from build123d import *

# Parameters (mm, degrees)
F1_DEPTH  = 5.2959
F2_DEPTH  = 41.276
F4_DEPTH  = 3.7084
F12_DEPTH = 3.7084
F6_DEPTH  = 10.5918
F7_DEPTH  = 41.276
F8_W      = 3.5700032353
F8_H      = 0.1361034085
F8_H_2    = 4.0928895229
F8_H_3    = 0.1088827268
F8_H_4    = 4.1201102046
F8_H_5    = 0.0816620451
F8_H_6    = 4.1473308863
F8_H_7    = 0.0544413634
F8_H_8    = 4.174551568
F8_H_9    = 0.0272206817
F8_H_10   = 4.2017722497
F8_H_11   = 4.2289929314
F14_DEPTH = 12.7
F9_R      = 1.016


with BuildPart() as f1:
    # F0 (on Right) → F1 (new body, symmetric)
    with BuildSketch(Plane.YZ):
        Polygon((25.4, 38.1), (0, 0), (41.275, 0), (41.275, 7.9375), (25.4, 15.875), align=None)
    extrude(amount=F1_DEPTH, both=True)

    # F10 (on Front) → F2 (cut, through all)
    with BuildSketch(Plane.XZ):
        with BuildLine():
            Line((-1.5875, 14.8209), (-5.2959, 14.8209))
            Line((-5.2959, 14.8209), (-5.2959, 5.2959000144))
            ThreePointArc((-5.2959, 5.2959000144), (-4.2692972482, 8.4295333251), (-1.5875, 10.3482658379))
            Line((-1.5875, 10.3482658379), (-1.5875, 14.8209))
        make_face()
        with BuildLine():
            Line((5.2959, 5.2959), (5.2959, 14.8209))
            Line((5.2959, 14.8209), (1.5875, 14.8209))
            Line((1.5875, 14.8209), (1.5875, 10.3482658379))
            ThreePointArc((1.5875, 10.3482658379), (4.2692972525, 8.4295333193), (5.2959, 5.2959))
        make_face()
        with BuildLine():
            ThreePointArc((0, 0), (-3.7447668076, 1.5511332026), (-5.2959, 5.2959000144))
            Line((-5.2959, 5.2959000144), (-5.2959, 0))
            Line((-5.2959, 0), (0, 0))
        make_face()
        with BuildLine():
            ThreePointArc((5.2959, 5.2959), (3.7447668025, 1.5511331975), (0, 0))
            Line((0, 0), (5.2959, 0))
            Line((5.2959, 0), (5.2959, 5.2959))
        make_face()
    extrude(amount=-F2_DEPTH, mode=Mode.SUBTRACT)

    # F3 (on face) → F4 (cut)
    with BuildSketch(Plane.YZ.offset(5.2959)):
        Polygon((17.4625, 14.8209), (27.5082, 14.8209), (25.4, 15.875), (25.4, 19.5834), align=None)
    extrude(amount=-F4_DEPTH, mode=Mode.SUBTRACT)

    # F11 (on face) → F12 (cut)
    with BuildSketch(Plane(origin=(-5.2959, 0, 0), x_dir=(0, -1, 0), z_dir=(-1, 0, 0))):
        Polygon((-27.5082, 14.8209), (-17.4625, 14.8209), (-25.4, 19.5834), (-25.4, 15.875), align=None)
    extrude(amount=-F12_DEPTH, mode=Mode.SUBTRACT)

    # F5 (on face) → F6 (join)
    with BuildSketch(Plane.YZ.offset(5.2959)):
        with BuildLine():
            add(Edge.make_bspline(
                [(9.8806, 14.8209), (9.7887178245, 17.0000575052), (7.8190504565, 20.9662638554), (18.9792610557, 30.802658642), (25.4, 38.1)],
                knots=[0, 0, 0, 0, 0.3217761524, 1, 1, 1, 1], degree=3))
            Line((9.8806, 14.8209), (25.4, 38.1))
        make_face()
    extrude(amount=-F6_DEPTH)

    # F13 (on Front) → F7 (cut, through all)
    with BuildSketch(Plane.XZ):
        with BuildLine():
            add(Edge.make_bspline(
                [(-5.2959, 14.8209), (-5.2959, 15.5472858351), (-5.2959, 17.5957404535), (-5.2959, 22.9229933342), (-5.2959, 29.9563074991), (-5.2959, 35.6675528807), (-5.2959, 38.1)],
                knots=[0, 0, 0, 0, 2.1791575052, 6.1453638554, 15.981758642, 23.2791, 23.2791, 23.2791, 23.2791], degree=3))
            Line((-5.2959, 14.8209), (-2.38125, 38.1))
            Line((-2.38125, 38.1), (-5.2959, 38.1))
        make_face()
        with BuildLine():
            Line((2.38125, 38.1), (5.2959, 14.8209))
            add(Edge.make_bspline(
                [(5.2959, 14.8209), (5.2959, 15.5472858351), (5.2959, 17.5957404535), (5.2959, 22.9229933342), (5.2959, 29.9563074991), (5.2959, 35.6675528807), (5.2959, 38.1)],
                knots=[0, 0, 0, 0, 2.1791575052, 6.1453638554, 15.981758642, 23.2791, 23.2791, 23.2791, 23.2791], degree=3))
            Line((5.2959, 38.1), (2.38125, 38.1))
        make_face()
    extrude(amount=-F7_DEPTH, mode=Mode.SUBTRACT)

    # F8 (on Right) → F14 (cut, symmetric)
    with BuildSketch(Plane.YZ):
        Polygon((3.1753500641, -0.1633240902), (3.1753500641, 0), (3.1753500641, 4.0656688412), (-0.3946531713, 4.0656688412), (-0.3946531713, -0.1633240902), align=None)
        with Locations((7.7402901024, -0.0680517042)):
            Rectangle(F8_W, F8_H)
        with Locations((7.7402901024, 2.0464447615)):
            Rectangle(F8_W, F8_H_2)
        with Locations((14.0902317584, -0.0544413634)):
            Rectangle(F8_W, F8_H_3)
        with Locations((14.0902317584, 2.0600551023)):
            Rectangle(F8_W, F8_H_4)
        with Locations((20.4401734144, -0.0408310225)):
            Rectangle(F8_W, F8_H_5)
        with Locations((20.4401734144, 2.0736654432)):
            Rectangle(F8_W, F8_H_6)
        with Locations((26.7901150703, -0.0272206817)):
            Rectangle(F8_W, F8_H_7)
        with Locations((26.7901150703, 2.087275784)):
            Rectangle(F8_W, F8_H_8)
        with Locations((33.1400567263, -0.0136103408)):
            Rectangle(F8_W, F8_H_9)
        with Locations((33.1400567263, 2.1008861249)):
            Rectangle(F8_W, F8_H_10)
        with Locations((39.4899983823, 2.1144964657)):
            Rectangle(F8_W, F8_H_11)
    extrude(amount=F14_DEPTH, both=True, mode=Mode.SUBTRACT)

    # F9
    f9_edges = [f1.edges().sort_by_distance(p)[0] for p in [
        (3.714975, 15.399413, 27.447632),
        (-3.714975, 15.399413, 27.447632),
    ]]
    fillet(f9_edges, radius=F9_R)


solid = f1.part
Geometry check sheet. Reference: the model listing, model coordinates, mm. A direction names the side the tool comes from. Coordinates: 2 decimals unless noted, no trailing zeros. Order: outer loops, then holes, each group sorted by start corner. A loop starts at its lowest first (then second) coordinate and runs counter-clockwise, first axis right, second up. Notation, with made-up numbers: (-34.75, -4) - (-21.75, -4) arc R25 ccw to (-21.75, 13) - close; hole circle Ø9 at (77.25, 25.25). An arc over 180 degrees is marked (long way). Answer in a Markdown table with one row per item. Add a question column.
1) Cross-section at A-A, the plane y = 8.5. Record the cut outline in (x, z), then the cut area to 3 significant figures.
2) Cross-section at B-B, the plane y = 26.5. Record the cut outline in (x, z) (1 decimal), then the cut area to 3 significant figures.
3) Release check for a two-part mould opening along Z. For faces 5 (the flat face through (0, 25.4, 27)), 6 (the flat face through (3.468, 21.487, 17.235)), 7 (the flat face through (4.21, 19.51, 23.48)) record: +Z half, -Z half, draft (parallel to the pull), parting line (faces both ways), or undercut.
4) Cross-section at C-C, the plane z = 9. Record the cut outline in (x, y) (3 decimals), then the cut area to 3 significant figures.
5) Material ranges on line 1 along Y through (x, z) = (0, 3) (3 decimals); line 2 along Z through (x, y) = (-3, 17); line 3 along Z through (x, y) = (-1.75, 10), recorded low to high. Write a range as [from, to].
6) Cross-section at D-D, the plane z = 14. Record the cut outline in (x, y), then the cut area to 3 significant figures.
7) Gauge pin test, flat ends, axial feed: P1, Ø4, axis at x = -4, z = 33, coming from the -Y side; P2, Ø3.5, axis at x = 2, z = 1.5, coming from the +Y side (3 decimals); P3, Ø10, axis at y = 13, z = 26, coming from the +X side; P4, Ø1.5, axis at y = 35, z = 14, coming from the -X side. Record the tip position at first contact, or that the pin passes through.
8) Set-up check for faces 1 (the flat face through (-1.588, 21, 13)), 2 (the flat face through (1.588, 21, 13)), 3 (the flat face through (0, 3.175, 2)), 4 (the flat face through (0, 18.655, 3)): record each of +Z, -Z, +X, -X, +Y, -Y from which the full face is reachable in a straight line by a thin tool's end or side.
Check result:
| question | item | result |
|---|---|---|
| 1 | outline | (-5.16, 4.09) - (5.16, 4.09) arc R5.3 ccw to (1.59, 10.35) - (1.59, 12.75) - (-1.59, 12.75) - (-1.59, 10.35) arc R5.3 ccw to start |
| 1 | area | 63.8 mm² |
| 2 | outline | (-5.2, 4.2) - (5.2, 4.2) arc R5.3 ccw to (1.6, 10.3) - (1.6, 15.3) - (-1.6, 15.3) - (-1.6, 10.3) arc R5.3 ccw to start |
| 2 | area | 71.1 mm² |
| 3 | face 5 | draft |
| 3 | face 6 | undercut |
| 3 | face 7 | +Z half |
| 4 | outline | (-3.785, 6) - (3.785, 6) - (3.785, 39.15) - (-3.785, 39.15) - close |
| 4 | area | 251 mm² |
| 5 | line 1 | y = [3.175, 5.955], [9.525, 12.305], [15.875, 18.655], [22.225, 25.005], [28.575, 31.355], [34.925, 37.705] |
| 5 | line 2 | z = [0.93, 9.66], [14.82, 29.01] |
| 5 | line 3 | z = [0.3, 10.29], [14.82, 20.45] |
| 6 | outline | (-1.59, 9.33) - (1.59, 9.33) - (1.59, 29.15) - (-1.59, 29.15) - close |
| 6 | area | 62.9 mm² |
| 7 | P1 | stops at y = 19.36 |
| 7 | P2 | stops at y = 37.705 |
| 7 | P3 | stops at x = 4.52 |
| 7 | P4 | passes through |
| 8 | face 1 | -X, +Y |
| 8 | face 2 | +X, +Y |
| 8 | face 3 | -Z, +X, -X, -Y |
| 8 | face 4 | -Z, +X, -X |
